from build123d import *

# Parameters (mm, degrees)
SKETCH1_W           = 52
SKETCH1_H           = 148.75
SKETCH1_R           = 2.75
SKETCH1_W_2         = 22
SKETCH1_H_2         = 80
BOSS_EXTRUDE2_DEPTH = 5
BOSS_EXTRUDE3_DEPTH = 30
BOSS_EXTRUDE5_DEPTH = 30
SKETCH3_R           = 2.5
CUT_EXTRUDE1_DEPTH  = 5
CUT_EXTRUDE2_REACH  = 252.438
SKETCH5_R           = 2.5
SKETCH6_W           = 15
SKETCH6_H           = 88.75
BOSS_EXTRUDE6_DEPTH = 5
FILLET1_R           = 5
FILLET2_R           = 5


with BuildPart() as part:
    # Sketch1 → Boss-Extrude2 (new body)
    with BuildSketch(Plane(origin=(0, 0, 0), x_dir=(1, 0, 0), z_dir=(0, 1, 0))):
        with Locations((26, 74.375)):
            Rectangle(SKETCH1_W, SKETCH1_H)
        with Locations(Location((10, 28.75, 0), (0, 0, 270))):
            Circle(SKETCH1_R, mode=Mode.SUBTRACT)
        with Locations(Location((42, 28.75, 0), (0, 0, 270))):
            Circle(SKETCH1_R, mode=Mode.SUBTRACT)
        with Locations(Location((10, 138.75, 0), (0, 0, 270))):
            Circle(SKETCH1_R, mode=Mode.SUBTRACT)
        with Locations(Location((42, 138.75, 0), (0, 0, 270))):
            Circle(SKETCH1_R, mode=Mode.SUBTRACT)
        with Locations((26, 78.75)):
            Rectangle(SKETCH1_W_2, SKETCH1_H_2, mode=Mode.SUBTRACT)
    extrude(amount=BOSS_EXTRUDE2_DEPTH)

    # Sketch2 → Boss-Extrude3 (add)
    with BuildSketch(Plane.XY):
        Polygon((0, 5), (0, 0), (2.071067812, 0), (-17.428932188, -19.5), (-74, -19.5), (-74, -14.5), (-19.5, -14.5), align=None)
        Polygon((71.5, -14.5), (122.5, -14.5), (122.5, -19.5), (69.428932188, -19.5), (49.928932188, 0), (52, 0), (52, 5), align=None)
    extrude(amount=-BOSS_EXTRUDE3_DEPTH)

    # Sketch4 → Boss-Extrude5 (add)
    with BuildSketch(Plane(origin=(0, 0, -148.75), x_dir=(-1, 0, 0), z_dir=(0, 0, -1))):
        Polygon((74, -14.5), (74, -44.5), (69, -44.5), (69, -19.5), (62.5, -19.5), (62.5, -44.5), (57.428932188, -44.5), (57.428932188, -19.5), (17.428932188, -19.5), (-2.071067812, 0), (0, 0), (0, 5), (19.5, -14.5), align=None)
    extrude(amount=-BOSS_EXTRUDE5_DEPTH)

    # Sketch3 → Cut-Extrude1 (cut)
    with BuildSketch(Plane(origin=(0, -14.5, 0), x_dir=(1, 0, 0), z_dir=(0, 1, 0))):
        with Locations(Location((-40.5, 15, 0), (0, 0, 180))):
            Circle(SKETCH3_R)
        with Locations(Location((112.5, 15, 0), (0, 0, 180))):
            Circle(SKETCH3_R)
    extrude(amount=-CUT_EXTRUDE1_DEPTH, mode=Mode.SUBTRACT)

    # Cut-Extrude2: up to this face of the body (flat: up to its plane)
    cut_extrude2_end = Plane(part.part.faces().sort_by_distance((-57.428932188, -32, -133.75))[0])
    # Sketch5 → Cut-Extrude2 (cut, up to the picked face)
    with BuildSketch(Plane.ZY.offset(74), mode=Mode.PRIVATE) as cut_extrude2_sk1:
        with Locations((-133.75, -32)):
            Circle(SKETCH5_R)
    cut_extrude2_tool1 = split(extrude(cut_extrude2_sk1.sketch, amount=-CUT_EXTRUDE2_REACH, mode=Mode.PRIVATE), bisect_by=cut_extrude2_end, keep=Keep.BOTH, mode=Mode.PRIVATE)
    add(cut_extrude2_tool1.solids().sort_by(Axis((-74, -32, -133.75), (1, 0, 0)))[0], mode=Mode.SUBTRACT)

    # Sketch6 → Boss-Extrude6 (add)
    with BuildSketch(Plane(origin=(0, -14.5, 0), x_dir=(1, 0, 0), z_dir=(0, 1, 0))):
        with Locations((-66.5, 74.375)):
            Rectangle(SKETCH6_W, SKETCH6_H)
    extrude(amount=-BOSS_EXTRUDE6_DEPTH)

    # Fillet1
    # the kernel refuses this fillet: 5 mm, written as the material it adds along each edge
    with BuildSketch(Plane(origin=(-59, -14.5, -118.75), x_dir=(0, 0, 1), z_dir=(0, -1, 0)), Plane(origin=(-59, -14.5, -30), x_dir=(1, 0, 0), z_dir=(0, -1, 0)), Plane(origin=(15, 0, -118.75), x_dir=(1, 0, 0), z_dir=(0, 1, 0))) as fillet1_piece_1:
        with BuildLine():
            CenterArc((FILLET1_R, -FILLET1_R), FILLET1_R, 90, 90)
            Line((0, -FILLET1_R), (0, 0))
            Line((0, 0), (FILLET1_R, 0))
        make_face()
    extrude(amount=5)
    with BuildSketch(Plane(origin=(15, 0, -38.75), x_dir=(1, 0, 0), z_dir=(0, 1, 0)), Plane(origin=(37, 0, -38.75), x_dir=(0, 0, -1), z_dir=(0, 1, 0)), Plane(origin=(37, 0, -118.75), x_dir=(-1, 0, 0), z_dir=(0, 1, 0))) as fillet1_piece_2:
        with BuildLine():
            CenterArc((FILLET1_R, FILLET1_R), FILLET1_R, 180, 90)
            Line((0, FILLET1_R), (0, 0))
            Line((0, 0), (FILLET1_R, 0))
        make_face()
    extrude(amount=5)
    # the kernel refuses this fillet: 5 mm, written as the material it takes off along each edge
    with BuildSketch(Plane(origin=(-74, -32, 0), x_dir=(1, 0, 0), z_dir=(0, 1, 0)), Plane(origin=(122.5, -2, 0), x_dir=(-1, 0, 0), z_dir=(0, -1, 0)), Plane(origin=(52, -12.5, -148.75), x_dir=(-1, 0, 0), z_dir=(0, 1, 0)), Plane(origin=(-86.5, -44.5, -148.75), x_dir=(0, 1, 0), z_dir=(1, 0, 0))) as fillet1_2_piece_1:
        with BuildLine():
            CenterArc((FILLET1_R, FILLET1_R), FILLET1_R, 180, 90)
            Line((0, FILLET1_R), (0, 0))
            Line((0, 0), (FILLET1_R, 0))
        make_face()
    extrude(amount=30, mode=Mode.SUBTRACT)
    with BuildSketch(Plane(origin=(122.5, -2, -30), x_dir=(-1, 0, 0), z_dir=(0, -1, 0)), Plane(origin=(-86.5, -44.5, -118.75), x_dir=(0, 1, 0), z_dir=(1, 0, 0))) as fillet1_2_piece_2:
        with BuildLine():
            CenterArc((FILLET1_R, -FILLET1_R), FILLET1_R, 90, 90)
            Line((0, -FILLET1_R), (0, 0))
            Line((0, 0), (FILLET1_R, 0))
        make_face()
    extrude(amount=30, mode=Mode.SUBTRACT)
    with BuildSketch(Plane(origin=(-75, -44.5, -118.75), x_dir=(0, 1, 0), z_dir=(1, 0, 0))) as fillet1_2_piece_3:
        with BuildLine():
            CenterArc((FILLET1_R, -FILLET1_R), FILLET1_R, 90, 90)
            Line((0, -FILLET1_R), (0, 0))
            Line((0, 0), (FILLET1_R, 0))
        make_face()
    extrude(amount=30.071067812, mode=Mode.SUBTRACT)
    with BuildSketch(Plane(origin=(-75, -44.5, -148.75), x_dir=(0, 1, 0), z_dir=(1, 0, 0))) as fillet1_2_piece_4:
        with BuildLine():
            CenterArc((FILLET1_R, FILLET1_R), FILLET1_R, 180, 90)
            Line((0, FILLET1_R), (0, 0))
            Line((0, 0), (FILLET1_R, 0))
        make_face()
    extrude(amount=30.071067812, mode=Mode.SUBTRACT)

    # Fillet2
    fillet2_edges = [part.edges().sort_by_distance(p)[0] for p in [
        (-19.5, -14.5, -15),
        (2.071067812, 0, -15),
        (-17.428932188, -19.5, -15),
        (49.928932188, 0, -15),
        (71.5, -14.5, -15),
        (69.428932188, -19.5, -15),
        (-19.5, -14.5, -133.75),
        (-17.428932188, -19.5, -133.75),
        (2.071067812, 0, -133.75),
    ]]
    fillet(fillet2_edges, radius=FILLET2_R)


solid = part.part
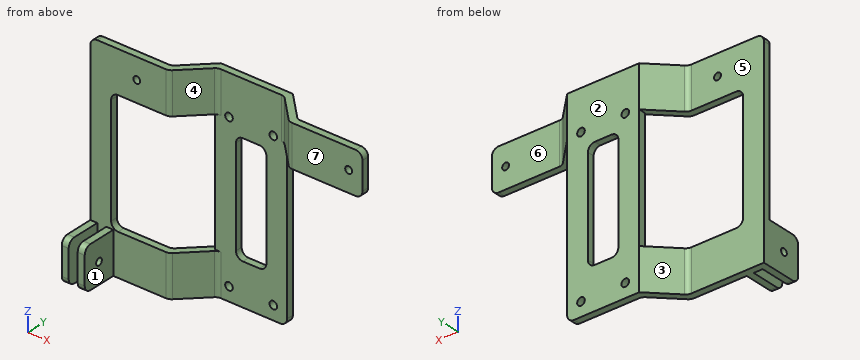
Verification items for the finished model (mm, model axes). Face numbers are marked on the shaded views. A direction names the side the tool comes from. Coordinates: 2 decimals unless noted, no trailing zeros. Write each loop counter-clockwise with the first axis right and the second up, starting at its lowest first coordinate (ties: lowest second). Pieces come first, ordered by that corner, then holes. Notation, with made-up numbers: (-26, 33) -> (3, 33) arc R26 ccw to (3, 52) -> close; hole circle Ø11 at (-14.75, 2.5). An arc over 180 degrees is marked (long way). One line per item, written item: value. Start each with the question number.
Q1. Cross-section at D-D on x = 42. Enter the section's corners in (y, z), and give its area (3 significant figures).
Q2. Thickness scan on L1, parallel to Z at x = -40.5, y = -16.9; L2, parallel to Y at x = -72.9, z = -133.75; L3, parallel to X at y = 3.5, z = -68.5. Record the ranges inside material, lowest first. Write a range as from..to.
Q3. Cross-section at A-A on z = -138.75. Enter the section's corners in (x, y).
Q4. Access from +Z, -Z, +X, -X, +Y, -Y to the whole of each face (thin tool, end or side, straight path). Record for the marked faces 5, 6 and 7.
Q5. Go/stop test with flat-tipped pins: P1, Ø7.5, axis at y = -36, z = -128, coming from the +X side; P2, Ø2.5, axis at y = -16, z = -57, coming from the +X side; P3, Ø9, axis at x = 89.5, z = -13.5, coming from the -Y side. Record where each tip stops, or that it passes through.
Q6. Cross-section at B-B on x = 112.5. Enter the section's corners in (y, z).
Q7. Cross-section at C-C on y = -24. Enter the section's corners in (x, z), and give its area (3 significant figures).
Q8. Mould release check, pull along X, two halves, no side actions. Record for the marked faces 1, 2, 3 and 4: pulls with the +X half, pulls with the -X half, needs draft (parallel to the pull), parting line crosses it, or undercut.
Checked values:
1. outline: (0, -148.75) -> (5, -148.75) -> (5, -141.5) -> (0, -141.5) -> close; (0, -136) -> (5, -136) -> (5, -31.5) -> (0, -31.5) -> close; (0, -26) -> (5, -26) -> (5, 0) -> (0, 0) -> close
1. area: 689 mm²
2. L1: z = -148.75..-118.75, -30..-17.5, -12.5..0
2. L2: y = -44.5..-34.5, -29.5..-14.5
2. L3: x = 0..15, 37..52
3. outline: (-74, -44.5) -> (-69, -44.5) -> (-69, -19.5) -> (-62.5, -19.5) -> (-62.5, -44.5) -> (-57.43, -44.5) -> (-57.43, -19.5) -> (-19.5, -19.5) arc R5 ccw to (-15.96, -18.04) -> (0.61, -1.46) arc R5 cw to (4.14, 0) -> (7.25, 0) -> (7.25, 5) -> (0, 5) -> (-18.04, -13.04) arc R5 cw to (-21.57, -14.5) -> (-74, -14.5) -> close; (12.75, 0) -> (39.25, 0) -> (39.25, 5) -> (12.75, 5) -> close; (44.75, 0) -> (52, 0) -> (52, 5) -> (44.75, 5) -> close
4. face 5: +Z, -Z, -X, +Y
4. face 6: +Z, -Z, +X, +Y
4. face 7: +Z, -Z, +X, -X, -Y
5. P1: stops at x = -57.43
5. P2: stops at x = -59
5. P3: stops at y = -19.5
6. outline: (-19.5, -30) -> (-14.5, -30) -> (-14.5, -17.5) -> (-19.5, -17.5) -> close; (-19.5, -12.5) -> (-14.5, -12.5) -> (-14.5, 0) -> (-19.5, 0) -> close
7. outline: (-74, -148.75) -> (-69, -148.75) -> (-69, -118.75) -> (-74, -118.75) -> close; (-62.5, -148.75) -> (-57.43, -148.75) -> (-57.43, -118.75) -> (-62.5, -118.75) -> close
7. area: 302 mm²
8. face 1: pulls with the +X half
8. face 2: needs draft
8. face 3: pulls with the -X half
8. face 4: undercut
